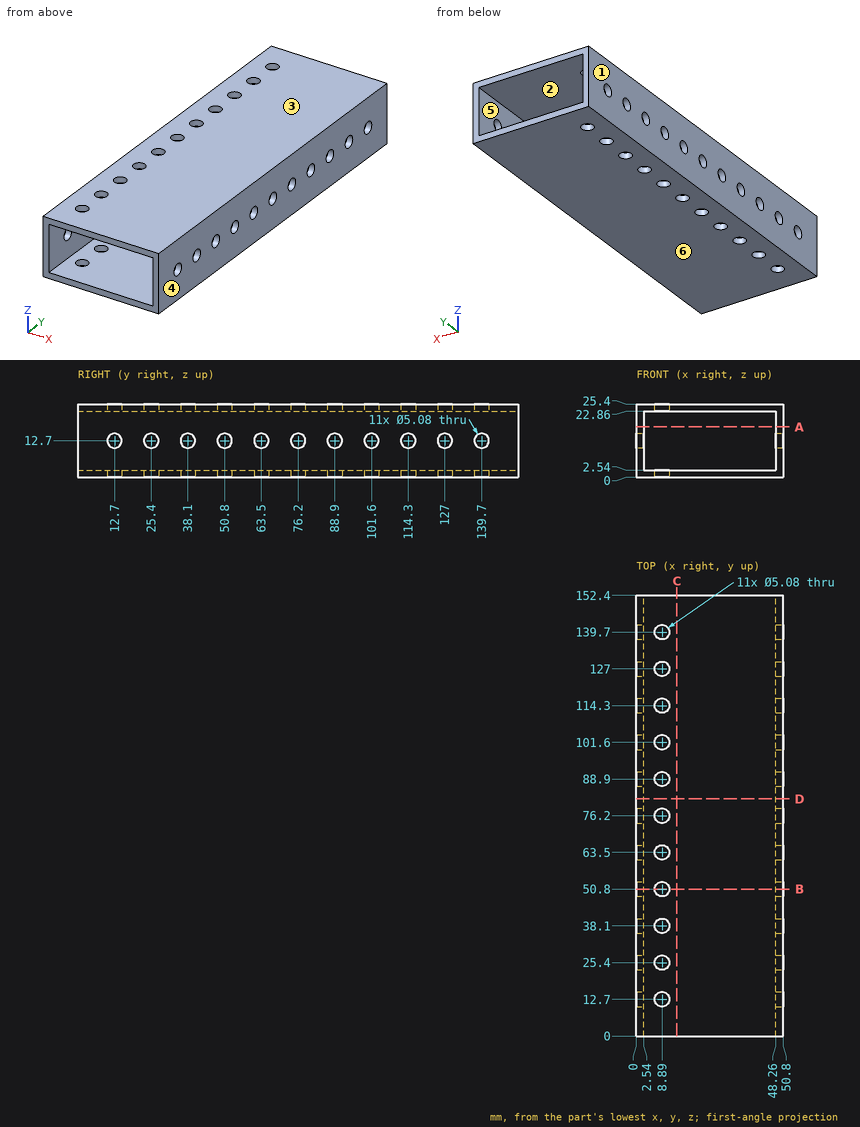
The drawing under review shows one solid part. Ordinate dimensions are in mm from its lowest x, y, z. A direction names the side the tool comes from. Give positions to 0.01 mm unless a question says otherwise; leave off trailing zeros. Write each loop counter-clockwise with the first axis right and the second up, starting at its lowest first coordinate (ties: lowest second). Pieces come first, ordered by that corner, then holes. Notation, with made-up numbers: M 16.5,31 L 53.5,31 A19 cw 53.5,51 Z; hole C 67.25,88.25 d10. An arc over 180 degrees is marked long. Write each question's results on one line, items separated by ' | '. Start each with the question number.
1. We need section A-A (z = 17.5). Write out the cut boundary in (x, y).
2. We need section B-B (y = 50.8). Write out the cut boundary in (x, z).
3. For the marked faces 5 and 6, list the 3-axis set-ups (+Z, -Z, +X, -X, +Y, -Y) from which the entire face can be reached by the end or side of a thin tool; tool diameter is ignored.
4. For probe 1 along Z at (x, y) = (31, 110); probe 2 along X at (y, z) = (88.5, 23.5); probe 3 along Z at (x, y) = (1, 114), list the stretches that pass through material, from the lowest coordinate up. Write a range as [from, to].
5. We need section D-D (y = 82). Write out the cut boundary in (x, z).
6. We need section C-C (x = 14). Write out the cut boundary in (y, z), and give its area (3 significant figures).
7. Mouldability with a two-part tool opening along X and no side actions: class the marked faces 1, 2, 3 and 4 as released by +X, released by -X, zero draft, split by the parting line, or undercut.
Results found:
1) outline: M 0,0 L 2.54,0 L 2.54,152.4 L 0,152.4 Z; M 48.26,0 L 50.8,0 L 50.8,152.4 L 48.26,152.4 Z
2) outline: M 0,0 L 6.35,0 L 6.35,2.54 L 2.54,2.54 L 2.54,10.16 L 0,10.16 Z; M 0,15.24 L 2.54,15.24 L 2.54,22.86 L 6.35,22.86 L 6.35,25.4 L 0,25.4 Z; M 11.43,0 L 50.8,0 L 50.8,10.16 L 48.26,10.16 L 48.26,2.54 L 11.43,2.54 Z; M 11.43,22.86 L 48.26,22.86 L 48.26,15.24 L 50.8,15.24 L 50.8,25.4 L 11.43,25.4 Z
3) face 5: +Y, -Y | face 6: -Z, +X, -X, +Y, -Y
4) probe 1: z = [0, 2.54], [22.86, 25.4] | probe 2: x = [0, 6.38], [11.4, 50.8] | probe 3: z = [0, 10.18], [15.22, 25.4]
5) outline: M 0,0 L 50.8,0 L 50.8,25.4 L 0,25.4 Z; hole M 2.54,2.54 L 48.26,2.54 L 48.26,22.86 L 2.54,22.86 Z
6) outline: M 0,0 L 152.4,0 L 152.4,2.54 L 0,2.54 Z; M 0,22.86 L 152.4,22.86 L 152.4,25.4 L 0,25.4 Z | area: 774 mm^2
7) face 1: released by -X | face 2: undercut | face 3: zero draft | face 4: released by +X
